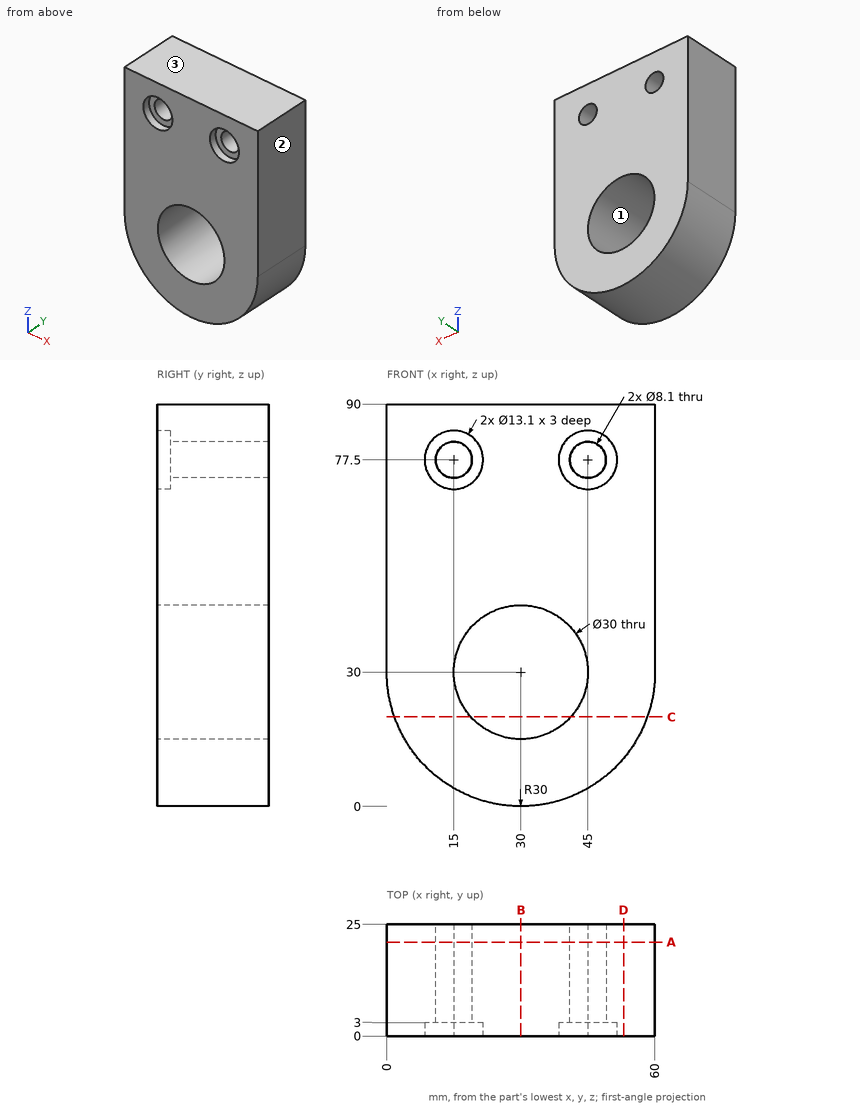
Could you check a few things on this drawing? It's one solid part, dimensions in mm from its lowest x, y, z. Give positions to 0.01 mm unless a question says otherwise; leave off trailing zeros. Write each loop counter-clockwise with the first axis right and the second up, starting at its lowest first coordinate (ties: lowest second). Pieces come first, ordered by that corner, then holes. Notation, with made-up numbers: (2, 9) -> (55, 9) arc R17 cw to (55, 26) -> close; hole circle Ø6 at (56, 32). An arc over 180 degrees is marked (long way). Answer as CSV lines item,"result". Start each with the question number.
(1) If we section it at D-D, the plane x = 53: Write out the boundary of the cut face in (y, z).
(2) If we mould it in two halves opening along Z, with no side actions, what happens to the marked faces 1, 2 and 3? For each: +Z half, -Z half, draft (parallel to the pull), parting line (faces both ways), or undercut.
(3) If we section it at A-A, the plane y = 21: Write out the boundary of the cut face in (x, z).
(4) If we section it at C-C, the plane z = 20: Write out the boundary of the cut face in (x, y), and give its area (3 significant figures).
(5) If we section it at B-B, the plane x = 30: Write out the boundary of the cut face in (y, z).
(6) Please list where these lines run through material, in increasing order: line 1 (X direction, y = 17, z = 77.5); line 2 (X direction, y = 10.75, z = 30.5); line 3 (Z direction, x = 36.5, y = 15.5).
(7) I'm going to push flat-ended pins straight in: pin 1 Ø10.5 at (x, z) = (15, 77.5) entering from +Y; pin 2 Ø1 at (x, y) = (47, 9.5) entering from -Z; pin 3 Ø2 at (x, y) = (18, 20) entering from -Z; pin 4 Ø4 at (x, y) = (45.5, 4.5) entering from -Z. Where does each tip first touch, or does it pass through?
Answer list:
1,outline,"(0, 10.74) -> (25, 10.74) -> (25, 90) -> (0, 90) -> close"
2,face 1,"undercut"
2,face 2,"draft"
2,face 3,"+Z half"
3,outline,"(0, 30) arc R30 ccw to (60, 30) -> (60, 90) -> (0, 90) -> close; hole circle Ø8.1 at (15, 77.5); hole circle Ø30 at (30, 30); hole circle Ø8.1 at (45, 77.5)"
4,outline,"(1.72, 0) -> (18.82, 0) -> (18.82, 25) -> (1.72, 25) -> close; (41.18, 0) -> (58.28, 0) -> (58.28, 25) -> (41.18, 25) -> close"
4,area,"855 mm^2"
5,outline,"(0, 0) -> (25, 0) -> (25, 15) -> (0, 15) -> close; (0, 45) -> (25, 45) -> (25, 90) -> (0, 90) -> close"
6,line 1,"0 to 10.95, 19.05 to 40.95, 49.05 to 60"
6,line 2,"0 to 15.01, 44.99 to 60"
6,line 3,"0.71 to 16.48, 43.52 to 90"
7,pin 1,"y = 25"
7,pin 2,"z = 4.95"
7,pin 3,"z = 2.09"
7,pin 4,"z = 3.21"
